Autodesk Inventor part; units mm, degrees
ref_plane "YZ Plane" through (0, 0, 0) normal (1, 0, 0) x (0, 1, 0)
ref_plane "XZ Plane" through (0, 0, 0) normal (0, 1, 0) x (-1, 0, 0)
ref_plane "XY Plane" through (0, 0, 0) normal (0, 0, 1) x (1, 0, 0)
sketch "Sketch1" plane through (0, 0, 0) normal (0, 0, 1) x (1, 0, 0)
  line L0 (0, 0) -> (0, 9.5) construction
  line L1 (0, 9.5) -> (3, 9.5)
  line L2 (3, 9.5) -> (3, 10.5)
  line L3 (3, 10.5) -> (3.5, 10.5)
  line L4 (3.5, 10.5) -> (3.5, 0) construction
  line L5 (3.5, 0) -> (0, 0) construction
  line L6 (0, 2.5) -> (3.5, 2.5)
  line L7 (3.5, 2.5) -> (3.5, 10.5)
  line L8 (0, 9.5) -> (-3, 9.5)
  line L9 (-3, 9.5) -> (-3, 10.5)
  line L10 (-3, 10.5) -> (-3.5, 10.5)
  line L11 (-3.5, 10.5) -> (-3.5, 0) construction
  line L12 (0, 2.5) -> (-3.5, 2.5)
  line L13 (-3.5, 2.5) -> (-3.5, 10.5)
  dimension "d0" = 2.5
  dimension "d1" = 3
  dimension "d2" = 0.5
  dimension "d8" = 1
  dimension "d10" = 10.5
revolve "Revolution2" add sketch "Sketch1" angle 360 about axis through (3.5, 0, 0) along (-1, 0, 0)
sketch "Sketch2" plane through (3.5, 0, 0) normal (1, 0, 0) x (0, 0, -1)
  circle A0 centre (0, 0) radius 2.5
  circle A1 centre (0, 6.5) radius 2
  dimension "d11" = 6.5
  dimension "d12" = 4
extrude "Extrusion1" cut sketch "Sketch2" against normal through all contours A1
pattern_circular "Circular Pattern1" count 3 over 360 about axis through (1.5, 0, 0) along (1, 0, 0) of "Extrusion1"
properties part number "FoilCoil"
Model file for the job. Use its own axes, mm. A direction names the side the tool comes from. Give positions to 0.01 mm unless a question says otherwise; leave off trailing zeros. Loops run counter-clockwise (first coordinate to the right, second up) from the corner with the lowest first, then second, coordinate; pieces in that order, holes last.
Item 1: Slice it at B-B (y = 0). Write the cut outline in (x, z), plus the area to 3 significant figures.
Check values:
outline: (-3.5, -10.5) - (-3, -10.5) - (-3, -9.5) - (3, -9.5) - (3, -10.5) - (3.5, -10.5) - (3.5, -2.5) - (-3.5, -2.5) - close; (-3.5, 2.5) - (3.5, 2.5) - (3.5, 10.5) - (3, 10.5) - (3, 9.5) - (-3, 9.5) - (-3, 10.5) - (-3.5, 10.5) - close
area: 100 mm2
Item 2: Slice it at D-D (y = -3.25). Write the cut outline in (x, z).
Check values:
outline: (-3.5, -9.98) - (-3, -9.98) - (-3, -8.93) - (3, -8.93) - (3, -9.98) - (3.5, -9.98) - (3.5, -7.63) - (-3.5, -7.63) - close; (-3.5, -3.63) - (3.5, -3.63) - (3.5, 3.63) - (-3.5, 3.63) - close; (-3.5, 7.63) - (3.5, 7.63) - (3.5, 9.98) - (3, 9.98) - (3, 8.93) - (-3, 8.93) - (-3, 9.98) - (-3.5, 9.98) - close
Item 3: Mould opens along Y. For faces 1 (the face through (0.049, -5.202, -5.196)), 2 (the face through (-3, -5, 9)), 3 (the face through (0.04, 4.38, -8.43)) say: +Y half, -Y half, draft (parallel to the pull), parting line (faces both ways), or undercut.
Check values:
face 1: undercut
face 2: draft
face 3: parting line
Item 4: Drill centre lines: line 1 along Y through (x, z) = (-0.75, 0); line 2 along Y through (x, z) = (3.25, 0); line 3 along X through (y, z) = (-7, -6.5). Where is each one in solid material? Low to high.
Check values:
line 1: y = -9.5 to -2.5, 2.5 to 4.5, 8.5 to 9.5
line 2: y = -10.5 to -2.5, 2.5 to 4.5, 8.5 to 10.5
line 3: x = -3.5 to -3, 3 to 3.5
Item 5: Which spindle directions (+Z, -Z, +X, -X, +Y, -Y) get a long thin tool onto all of the face, cutting with end or side? Do faces 4 (the face through (0.049, 8.483, 0.26)), 5 (the face through (3, -5, 9)). Say none if no direction does.
Check values:
face 4: +X, -X
face 5: none
Item 6: Drop flat-ended pins along their axis: P1, Ø3.5, axis at y = -3.25, z = 5.63, coming from the +X side; P2, Ø4, axis at x = -2, y = -4, coming from the +Z side. Give the stop position or say it passes through.
Check values:
P1: passes through
P2: stops at z = 10.25
Item 7: Slice it at C-C (z = 4.75). Write the cut outline in (x, y), plus the area to 3 significant figures.
Check values:
outline: (-3.5, -9.36) - (-3, -9.36) - (-3, -8.23) - (3, -8.23) - (3, -9.36) - (3.5, -9.36) - (3.5, -5.05) - (-3.5, -5.05) - close; (-3.5, -1.45) - (3.5, -1.45) - (3.5, 9.36) - (3, 9.36) - (3, 8.23) - (-3, 8.23) - (-3, 9.36) - (-3.5, 9.36) - close
area: 92.3 mm2
Item 8: Slice it at A-A (z = 0). Write the cut outline in (x, y).
Check values:
outline: (-3.5, -10.5) - (-3, -10.5) - (-3, -9.5) - (3, -9.5) - (3, -10.5) - (3.5, -10.5) - (3.5, -2.5) - (-3.5, -2.5) - close; (-3.5, 2.5) - (3.5, 2.5) - (3.5, 4.5) - (-3.5, 4.5) - close; (-3.5, 8.5) - (3.5, 8.5) - (3.5, 10.5) - (3, 10.5) - (3, 9.5) - (-3, 9.5) - (-3, 10.5) - (-3.5, 10.5) - close
